from build123d import *

# Parameters (mm, degrees)
F1_DEPTH = 5
F2_R     = 25
F3_DEPTH = 5
F6_R     = 7.5
F4_R     = 17.5
F8_R     = 5.5
F9_DEPTH = 40


with BuildPart() as f1:
    # F0 (on Top) → F1 (new body)
    with BuildSketch(Plane.XY):
        with BuildLine():
            Line((3, -4.609772), (3, -24.819347))
            ThreePointArc((3, -24.819347), (0, 25), (-3, -24.819347))
            Line((-3, -24.819347), (-3, -4.609772))
            Line((-3, -4.609772), (3, -4.609772))
        make_face()
    extrude(amount=F1_DEPTH)

    # F2 (on face) → F3 (join)
    with BuildSketch(Plane.XY.offset(5)):
        Circle(F2_R)
    extrude(amount=F3_DEPTH)

    # F6 (on offset) → F7 section 0
    with BuildSketch(Plane.XY.offset(40)):
        Circle(F6_R)
    # F4 (on face) → F7 section 1
    with BuildSketch(Plane.XY.offset(10)):
        Circle(F4_R)
    loft()

    # F8 (on face) → F9 (cut, through all)
    with BuildSketch(Plane.XY.offset(40)):
        Circle(F8_R)
    extrude(amount=-F9_DEPTH, mode=Mode.SUBTRACT)


solid = f1.part
Input: part model. Units: mm. Frame: model coordinates. A direction names the side the tool comes from. Coordinates: 2 decimals unless noted, no trailing zeros. Loops run counter-clockwise (first coordinate to the right, second up) from the corner with the lowest first, then second, coordinate; pieces in that order, holes last.
(1) First-contact query: pin 1 Ø1.5 at (x, z) = (4.5, 34) entering from -Y; pin 2 Ø5.5 at (y, z) = (-15.5, 3.5) entering from -X; pin 3 Ø10 at (y, z) = (12.5, 8.5) entering from -X. Flat tips, straight axial feed; report the tip coordinate or a pass-through.
(2) Material intervals for probe 1 along Z at (x, y) = (-2.5, 18); probe 2 along X at (y, z) = (0, 6); probe 3 along X at (y, z) = (-5, 12), sorted ascending.
(3) Section C-C on y = 21.5. Return the cut outline in (x, z), then the cut area to 3 significant figures.
(4) Set-up query: faces 1 (the face through (-17, -5, 10)), 2 (the face through (3, -15, 2)), 3 (the face through (-0.716, 5.453, 20.28)). Return all of +Z, -Z, +X, -X, +Y, -Y with unobstructed straight access to the full face (end or side cutting, diameter ignored); none if empty.
(5) Pull-direction query (X, two-part tool) for faces 4 (the face through (-4, 4, 40)), 5 (the face through (-3, -15, 2)), 6 (the face through (-2.48, -11.19, 28.12)); classes: released by +X, released by -X, zero draft, split by the parting line, or undercut.
(6) Section A-A on x = 0. Return the cut outline in (y, z), then the cut area to 4 significant figures.
(7) Section B-B on z = 8. Return the cut outline in (x, y).
Data:
1. pin 1: stops at y = -8.83
1. pin 2: stops at x = -21.5
1. pin 3: stops at x = -23.85
2. probe 1: z = 0 to 10
2. probe 2: x = -25 to -5.5, 5.5 to 25
2. probe 3: x = -16.07 to -2.29, 2.29 to 16.07
3. outline: (-12.76, 0) - (12.76, 0) - (12.76, 10) - (-12.76, 10) - close
3. area: 255 mm2
4. face 1: +Z
4. face 2: -Z, -Y
4. face 3: +Z, -Z
5. face 4: zero draft
5. face 5: undercut
5. face 6: split by the parting line
6. outline: (-25, 5) - (-5.5, 5) - (-5.5, 40) - (-7.5, 40) - (-17.5, 10) - (-25, 10) - close; (5.5, 0) - (25, 0) - (25, 10) - (17.5, 10) - (7.5, 40) - (5.5, 40) - close
6. area: 712.5 mm2
7. outline: circle Ø50 at (0, 0); hole circle Ø11 at (0, 0)
